Autodesk Fusion 360 part; units mm, degrees
sketch "Sketch1" plane through (0, 0, 0) normal (0, 1, 0) x (1, 0, 0)
  line L0 (0, 18) -> (35.7211, 18)
  line L1 (0, -18) -> (35.9683, -17.5009)
  arc A0 (35.7211, 18) -> (35.9683, -17.5009) centre (0, 0) ccw
  arc A1 (0, 18) -> (0.4995, -17.9931) centre (0, 0) ccw
  circle A2 centre (0, 28) radius 5
  circle A3 centre (0, -28) radius 5
  circle A4 centre (-28, 0) radius 5
  dimension "d1" = 80
  dimension "d2" = 36
  dimension "d4" = 28
  dimension "d5" = 28
  dimension "d6" = 28
  dimension "d7" = 10
  dimension "d8" = 10
  dimension "d9" = 10
extrude "Extrude1" add sketch "Sketch1" along normal blind 5
The listing builds one solid part. Answer for the finished solid, in the listing's coordinates (mm). A direction names the side the tool comes from. Round coordinates to 2 decimals unless told otherwise and drop trailing zeros. Loops run counter-clockwise (first coordinate to the right, second up) from the corner with the lowest first, then second, coordinate; pieces in that order, holes last. Notation, with made-up numbers: (56, 49) -> (111, 49) arc R12 ccw to (111, 63) -> close; hole circle Ø9 at (13, -31). An arc over 180 degrees is marked (long way). Use one line per item in the form item = value.
1. The part is cut by section B-B on x = 27. Determine the outline of the cut face in (y, z).
Answer key:
outline = (0, -29.51) -> (5, -29.51) -> (5, -18) -> (0, -18) -> close; (0, 17.63) -> (5, 17.63) -> (5, 29.51) -> (0, 29.51) -> close
2. The part is cut by section A-A on y = 0.9. Determine the outline of the cut face in (x, z).
Answer key:
outline = (0, -18) arc R18 cw to (0, 18) -> (35.97, 17.5) arc R40 ccw (long way) to (35.72, -18) -> close; hole circle Ø10 at (-28, 0); hole circle Ø10 at (0, -28); hole circle Ø10 at (0, 28)
3. A tool of negligible diameter and unlimited length cuts with its end or side. For faces 1 (the cylindrical face through (-1.08, 2.46, -32.88)), 2 (the flat face through (18, 2, -18)), from which of +Z, -Z, +X, -X, +Y, -Y can it reach the whole face along a straight path? Write none if from no direction.
Answer key:
face_1 = +Y, -Y
face_2 = +X, +Y, -Y
4. For a pull along Z with two mould halves and no side action, classify faces 3 (the cylindrical face through (-1.08, 2.46, 23.12)), 4 (the flat face through (-19, 0, -1)), 5 (the cylindrical face through (-39.96, 2.46, 1.78)) as released by +Z, released by -Z, zero draft, split by the parting line, or undercut.
Answer key:
face_3 = undercut
face_4 = zero draft
face_5 = split by the parting line
5. Find the intervals of material crossed by probe 1 along Z at (x, y) = (0, 3.65); probe 2 along X at (y, z) = (3.15, 0); probe 3 along Z at (x, y) = (-31.5, 3.55), in increasing order. Write a range as [from, to].
Answer key:
probe_1 = [-40, -33], [-23, -18], [18, 23], [33, 40]
probe_2 = [-40, -33], [-23, -18]
probe_3 = [-24.65, -3.57], [3.57, 24.65]
6. The part is cut by section D-D on x = -3.5. Determine the outline of the cut face in (y, z), and give its area (3 significant figures).
Answer key:
outline = (0, -39.85) -> (5, -39.85) -> (5, -31.57) -> (0, -31.57) -> close; (0, -24.43) -> (5, -24.43) -> (5, -17.66) -> (0, -17.66) -> close; (0, 17.66) -> (5, 17.66) -> (5, 24.43) -> (0, 24.43) -> close; (0, 31.57) -> (5, 31.57) -> (5, 39.85) -> (0, 39.85) -> close
area = 150 mm²
7. Flat-ended cylindrical pins translate along their axes: pin 1 Ø2 at (y, z) = (1, 11) entering from +X; pin 2 Ø16 at (x, z) = (0, -28) entering from +Y; pin 3 Ø3 at (x, y) = (5.5, 3) entering from +Z. Find the tip coordinate at first contact, or state that the pin passes through.
Answer key:
pin_1 = -13.42
pin_2 = 5
pin_3 = 39.8
8. The part is cut by section C-C on z = -28. Determine the outline of the cut face in (x, y), and give its area (3 significant figures).
Answer key:
outline = (-28.57, 0) -> (-5, 0) -> (-5, 5) -> (-28.57, 5) -> close; (5, 0) -> (28.57, 0) -> (28.57, 5) -> (5, 5) -> close
area = 236 mm²
